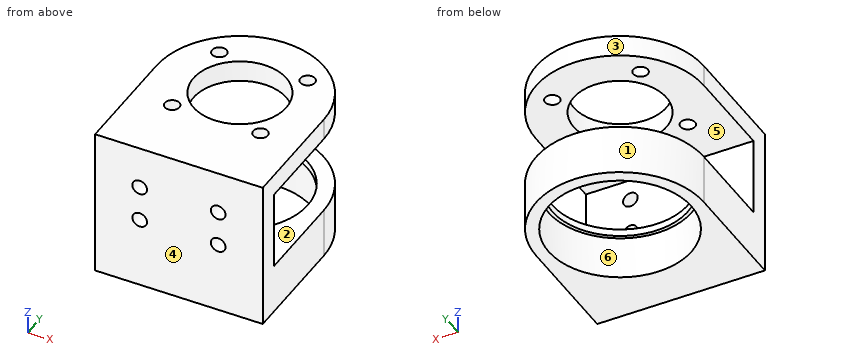
from build123d import *

# Parameters (mm, degrees)
EXTRUDE_1_DEPTH        = 36
SKETCH_3_R             = 13
CUT_EXTRUDE_1_DEPTH    = 20
HOLE_WIZARD_M4_1_D     = 4.1
HOLE_WIZARD_M4_1_DEPTH = 20
HOLE_WIZARD_M4_1_TIP   = 1.231764269
SKETCH_17_W            = 22
SKETCH_17_H            = 45.5
CUT_EXTRUDE_4_DEPTH    = 82.149553295
HOLE_WIZARD_M4_2_D     = 4.1
HOLE_WIZARD_M4_2_DEPTH = 10.1
HOLE_WIZARD_M4_2_TIP   = 1.231764269
SKETCH_21_R            = 20
CUT_EXTRUDE_5_DEPTH    = 6
SKETCH_22_R            = 19
CUT_EXTRUDE_6_DEPTH    = 10
SKETCH_26_W            = 47
SKETCH_26_H            = 22
CUT_EXTRUDE_8_DEPTH    = 4
EXTRUDE_START          = 6
SKETCH_27_R            = 20
EXTRUDE_2_DEPTH        = 6


with BuildPart() as part:
    # 草图2 → 凸台-拉伸1 (new body)
    with BuildSketch(Plane.XY):
        with BuildLine():
            Line((-23.5, 32), (-23.5, 0))
            Line((-23.5, 0), (23.5, 0))
            Line((23.5, 0), (23.5, 32))
            ThreePointArc((23.5, 32), (0, 55.5), (-23.5, 32))
        make_face()
    extrude(amount=EXTRUDE_1_DEPTH)

    # 草图3 → 切除-拉伸1 (cut)
    with BuildSketch(Plane.XY.offset(36)):
        with Locations((0, 32)):
            Circle(SKETCH_3_R)
    extrude(amount=-CUT_EXTRUDE_1_DEPTH, mode=Mode.SUBTRACT)

    # M4 间隙孔1
    with Locations(Plane.XY.offset(36)):
        with Locations((12.374368671, 19.625631329), (-12.374368671, 44.374368671), (12.374368671, 44.374368671), (-12.374368671, 19.625631329)):
            Hole(HOLE_WIZARD_M4_1_D / 2, depth=HOLE_WIZARD_M4_1_DEPTH)
            with Locations((0, 0, -(HOLE_WIZARD_M4_1_DEPTH + HOLE_WIZARD_M4_1_TIP / 2))):  # 118° drill point
                Cone(0, HOLE_WIZARD_M4_1_D / 2, HOLE_WIZARD_M4_1_TIP, mode=Mode.SUBTRACT)

    # 草图17 → 切除-拉伸4 (cut, through all)
    with BuildSketch(Plane(origin=(23.5, 0, 0), x_dir=(0, 0, -1), z_dir=(1, 0, 0))):
        with Locations((-19, 32.75)):
            Rectangle(SKETCH_17_W, SKETCH_17_H)
    extrude(amount=-CUT_EXTRUDE_4_DEPTH, mode=Mode.SUBTRACT)

    # M4 间隙孔2
    with Locations(Plane(origin=(0, 10, 0), x_dir=(1, 0, 0), z_dir=(0, 1, 0))):
        with Locations((-11, -14), (11, -14), (11, -24), (-11, -24)):
            Hole(HOLE_WIZARD_M4_2_D / 2, depth=HOLE_WIZARD_M4_2_DEPTH)
            with Locations((0, 0, -(HOLE_WIZARD_M4_2_DEPTH + HOLE_WIZARD_M4_2_TIP / 2))):  # 118° drill point
                Cone(0, HOLE_WIZARD_M4_2_D / 2, HOLE_WIZARD_M4_2_TIP, mode=Mode.SUBTRACT)

    # 草图21 → 切除-拉伸5 (cut)
    with BuildSketch(Plane(origin=(0, 0, 0), x_dir=(-1, 0, 0), z_dir=(0, 0, -1))):
        with Locations((0, 32)):
            Circle(SKETCH_21_R)
    extrude(amount=-CUT_EXTRUDE_5_DEPTH, mode=Mode.SUBTRACT)

    # 草图22 → 切除-拉伸6 (cut)
    with BuildSketch(Plane(origin=(0, 0, 6), x_dir=(-1, 0, 0), z_dir=(0, 0, -1))):
        with Locations((0, 32)):
            Circle(SKETCH_22_R)
    extrude(amount=-CUT_EXTRUDE_6_DEPTH, mode=Mode.SUBTRACT)

    # 草图26 → 切除-拉伸8 (cut)
    with BuildSketch(Plane(origin=(0, 10, 0), x_dir=(1, 0, 0), z_dir=(0, 1, 0))):
        with Locations((0, -19)):
            Rectangle(SKETCH_26_W, SKETCH_26_H)
    extrude(amount=-CUT_EXTRUDE_8_DEPTH, mode=Mode.SUBTRACT)

    # 草图27 → 凸台-拉伸2 (add)
    with BuildSketch(Plane(origin=(0, 0, 0), x_dir=(-1, 0, 0), z_dir=(0, 0, -1)).offset(EXTRUDE_START)):
        with BuildLine():
            Line((-23.5, 32), (-23.5, 0))
            Line((-23.5, 0), (23.5, 0))
            Line((23.5, 0), (23.5, 32))
            ThreePointArc((23.5, 32), (0, 55.5), (-23.5, 32))
        make_face()
        with Locations((0, 32)):
            Circle(SKETCH_27_R, mode=Mode.SUBTRACT)
    extrude(amount=-EXTRUDE_2_DEPTH)


solid = part.part
Geometry: final body of the model. Coordinates: model frame, mm. Face numbers are marked on the shaded views. A direction names the side the tool comes from. Give positions to 0.01 mm unless a question says otherwise; leave off trailing zeros. Write each loop counter-clockwise with the first axis right and the second up, starting at its lowest first coordinate (ties: lowest second). Pieces come first, ordered by that corner, then holes. Notation, with made-up numbers: (66.25, 25) -> (85.25, 25) arc R30 ccw to (85.25, 62) -> close; hole circle Ø6 at (62, 61.5). An arc over 180 degrees is marked (long way). Answer in a Markdown table with one row per item.
(1) Draft query along Y for the marked faces 3, 4, 5 and 6. Return one class per face: +Y half, -Y half, draft (parallel to the pull), parting line (faces both ways), or undercut.
Answers below:
| item | result |
|---|---|
| face 3 | +Y half |
| face 4 | -Y half |
| face 5 | draft |
| face 6 | undercut |
(2) Section query D-D on y = 29.5. Return loops of the section in (x, z), then the cut area to 3 significant figures.
Answers below:
| item | result |
|---|---|
| outline | (-23.5, -6) -> (-19.84, -6) -> (-19.84, 6) -> (-18.83, 6) -> (-18.83, 8) -> (-23.5, 8) -> close; (-23.5, 30) -> (-12.76, 30) -> (-12.76, 36) -> (-23.5, 36) -> close; (12.76, 30) -> (23.5, 30) -> (23.5, 36) -> (12.76, 36) -> close; (18.83, 6) -> (19.84, 6) -> (19.84, -6) -> (23.5, -6) -> (23.5, 8) -> (18.83, 8) -> close |
| area | 235 mm^2 |
(3) Section query B-B on y = 50. Return loops of the section in (x, z), then the cut area to 3 significant figures.
Answers below:
| item | result |
|---|---|
| outline | (-15.11, -6) -> (-8.72, -6) -> (-8.72, 6) -> (-6.08, 6) -> (-6.08, 8) -> (-15.11, 8) -> close; (-15.11, 30) -> (15.11, 30) -> (15.11, 36) -> (-15.11, 36) -> close; (6.08, 6) -> (8.72, 6) -> (8.72, -6) -> (15.11, -6) -> (15.11, 8) -> (6.08, 8) -> close |
| area | 371 mm^2 |
(4) Set-up query: the marked faces 1 and 2. Return all of +Z, -Z, +X, -X, +Y, -Y with unobstructed straight access to the full face (end or side cutting, diameter ignored); none if empty.
Answers below:
| item | result |
|---|---|
| face 1 | +Z, -Z, +Y |
| face 2 | +X, -X, +Y |
(5) Pin query (flat end, axial travel): pin 1 (3.5 mm diameter, centred on x = -12.37, y = 44.37, fed in from +Z); pin 2 (6.5 mm diameter, centred on x = 11, z = 24, fed in from +Y); pin 3 (17.5 mm diameter, centred on x = 11, z = 16.5, fed in from +Y). Return the tip coordinate at first contact, or that it passes through.
Answers below:
| item | result |
|---|---|
| pin 1 | z = 8 |
| pin 2 | y = 6 |
| pin 3 | y = 53.74 |
(6) Section query C-C on x = 18. Return loops of the section in (y, z).
Answers below:
| item | result |
|---|---|
| outline | (0, -6) -> (23.28, -6) -> (23.28, 6) -> (25.92, 6) -> (25.92, 8) -> (6, 8) -> (6, 30) -> (47.11, 30) -> (47.11, 36) -> (0, 36) -> close; (38.08, 6) -> (40.72, 6) -> (40.72, -6) -> (47.11, -6) -> (47.11, 8) -> (38.08, 8) -> close |
(7) Ray query, line 1 along Z through (x, y) = (11, 3.75); line 2 along X through (y, z) = (4.65, 24); line 3 along Z through (x, y) = (19, 30). Return the intervals inside material, ascending. Write a range as [from, to].
Answers below:
| item | result |
|---|---|
| line 1 | [-6, 11.95], [16.05, 21.95], [26.05, 36] |
| line 2 | [-23.5, -13.05], [-8.95, 8.95], [13.05, 23.5] |
| line 3 | [6, 8], [30, 36] |
(8) Section query A-A on x = 0. Return loops of the section in (y, z).
Answers below:
| item | result |
|---|---|
| outline | (0, -6) -> (12, -6) -> (12, 6) -> (13, 6) -> (13, 8) -> (6, 8) -> (6, 30) -> (19, 30) -> (19, 36) -> (0, 36) -> close; (45, 30) -> (55.5, 30) -> (55.5, 36) -> (45, 36) -> close; (51, 6) -> (52, 6) -> (52, -6) -> (55.5, -6) -> (55.5, 8) -> (51, 8) -> close |
